Could you check a few things on this model? Use its own coordinates, in mm. A direction names the side the tool comes from. Round coordinates to 2 decimals unless told otherwise and drop trailing zeros. Write each loop counter-clockwise with the first axis right and the second up, starting at its lowest first coordinate (ties: lowest second). Pieces come first, ordered by that corner, then holes. Notation, with made-up numbers: (57, 40.25) -> (86, 40.25) arc R24 cw to (86, 53.25) -> close; hole circle Ø3 at (81, 1.5). An arc over 180 degrees is marked (long way). One line per question, with ' | ' between items. Start each with the question number.
1. Imagine slicing it at A-A, the plane x = -71. List the corners of the cut face in (y, z) for me, and give its area (3 significant figures).
2. If I drill on line 1 along X through (y, z) = (18.75, 0); line 2 along X through (y, z) = (71, 0); line 3 along Z through (x, y) = (0, 57.5), over which ranges is the centre line in solid material (lowest first)? Write a range as [from, to].
3. For faces 1 (the flat face through (26, 30, -60)), 2 (the flat face through (0, 5, -95)), 3 (the flat face through (95, 5, 0)), 4 (the flat face through (-90, 5, -30)), which set-ups out of +Z, -Z, +X, -X, +Y, -Y let a thin tool reach every point of the face, with its end or its side?
4. For pin 1 Ø4 at (x, y) = (-22.5, 8.5) entering from +Z; pin 2 Ø1.5 at (x, y) = (54, 30.5) entering from -Z; pin 3 Ø11 at (x, y) = (88, 5) entering from -Z; pin 4 Ø4 at (x, z) = (76, 70) entering from +Y, each with a flat end and sliding along its axis, tell me the tip position at first contact or that it passes through.
5. Thinking about a two-plate mould opening in X: for faces 5 (the flat face through (30, 5, -90)), 6 (the flat face through (47.465, 4.93, -82.212)), 7 (the flat face through (94, 10, 15)), 8 (the conical face through (-10.03, 48.75, -45.15)), which applies, released by +X, released by -X, zero draft, split by the parting line, or undercut?
6. Imagine slicing it at C-C, the plane y = 44.5. List the corners of the cut face in (x, z) for me.
7. Imagine slicing it at B-B, the plane y = 17. List the corners of the cut face in (x, z) for me, and give its area (3 significant figures).
Autodesk Inventor part; units mm, degrees
ref_plane "YZ Plane" through (0, 0, 0) normal (1, 0, 0) x (0, 1, 0)
ref_plane "XZ Plane" through (0, 0, 0) normal (0, 1, 0) x (-1, 0, 0)
ref_plane "XY Plane" through (0, 0, 0) normal (0, 0, 1) x (1, 0, 0)
sketch "Sketch1" plane through (0, 0, 0) normal (0, 1, 0) x (-1, 0, 0)
  circle A0 centre (0, 0) radius 100
  dimension "d0" = 200
extrude "Extrusion1" add sketch "Sketch1" along normal blind 50
sketch "Sketch2" plane through (0, 0, 0) normal (0, -1, 0) x (1, 0, 0)
  circle A0 centre (0, 0) radius 90
  dimension "d3" = 180
extrude "Extrusion2" cut sketch "Sketch2" against normal blind 30
sketch "Sketch3" plane through (0, 0, 0) normal (1, 0, 0) x (0, 1, 0)
  line L0 (0, 0) -> (10, 0)
  line L1 (10, 0) -> (10, -30)
  line L2 (10, -30) -> (0, -30)
  line L3 (0, -30) -> (0, 0)
  dimension "d6" = 10
  dimension "d7" = 30
extrude "Extrusion3" cut sketch "Sketch3" against normal blind 400
pattern_circular "Circular Pattern1" count 12 over 360 about axis through (0, -10, 0) along (0, 1, 0) of "Extrusion3"
sketch "Sketch4" plane through (0, 50, 0) normal (0, 1, 0) x (1, 0, 0)
  circle A0 centre (0, 0) radius 60
  dimension "d13" = 120
extrude "Extrusion4" add sketch "Sketch4" along normal blind 30
sketch "Sketch5" plane through (0, 80, 0) normal (0, 1, 0) x (1, 0, 0)
  circle A0 centre (0, 0) radius 50
  dimension "d16" = 100
extrude "Extrusion5" cut sketch "Sketch5" against normal blind 20
sketch "Sketch6" plane through (0, 60, 0) normal (0, 1, 0) x (1, 0, 0)
  circle A0 centre (0, 0) radius 45
  dimension "d19" = 90
extrude "Extrusion6" cut sketch "Sketch6" against normal blind 50
chamfer "Chamfer1" distance 20 angle 45 1 edges at (-45, 30, 0)
properties part number "Slo"
Geometry results:
1) outline: (0, 55.31) -> (30, 55.31) -> (30, -55.31) -> (10, -55.31) -> (10, -70.42) -> (50, -70.42) -> (50, 70.42) -> (10, 70.42) -> (10, 62.98) -> (0, 62.98) -> close | area: 3,500 mm2
2) line 1: x = [-100, -90], [90, 100] | line 2: x = [-60, -50], [50, 60] | line 3: z = [-60, -45], [45, 60]
3) face 1: -Y | face 2: -Z, -Y | face 3: +X, -Y | face 4: +X, -X, -Y
4) pin 1: stops at z = 97.73 | pin 2: stops at z = -84.64 | pin 3: stops at z = -56.51 | pin 4: passes through
5) face 5: undercut | face 6: released by +X | face 7: zero draft | face 8: undercut
6) outline: circle Ø200 at (0, 0); hole circle Ø101 at (0, 0)
7) outline: circle Ø200 at (0, 0); hole circle Ø180 at (0, 0) | area: 5,970 mm2
